Source: CAD feature listing. Evaluate the final solid. Frame: model axes, mm. Face numbers are marked on the shaded views. A direction names the side the tool comes from. Coordinates: 2 decimals unless noted, no trailing zeros. Write each loop counter-clockwise with the first axis right and the second up, starting at its lowest first coordinate (ties: lowest second). Pieces come first, ordered by that corner, then holes. Notation, with made-up numbers: M -28.75,81 L -21.75,81 A20 cw -21.75,89 Z; hole C 85,-35 d8. An arc over 180 degrees is marked long. One line per item, written item: value. Start each with the question number.
Item 1: Cut plane A-A, the plane z = 8. Output: boundary loops of the cut face in (x, y).
Item 2: Mould query, pull axis Z, two halves, no side actions, for the marked faces 3, 4 and 5. Classes: released by +Z, released by -Z, zero draft, split by the parting line, or undercut.
Item 3: Cut plane D-D, the plane z = 30. Output: boundary loops of the cut face in (x, y), then the cut area to 3 significant figures.
Item 4: Cut plane C-C, the plane y = 1.75. Output: boundary loops of the cut face in (x, z), then the cut area to 3 significant figures.
Item 5: Cut plane B-B, the plane x = 64. Output: boundary loops of the cut face in (y, z), then the cut area to 3 significant figures.
Item 6: Set-up query: the marked faces 1 and 2. Return all of +Z, -Z, +X, -X, +Y, -Y with unobstructed straight access to the full face (end or side cutting, diameter ignored); none if empty.
Item 7: Pin query (flat end, axial travel): P1, Ø6, axis at x = 19, z = 32, coming from the +Y side; P2, Ø8, axis at x = 6, z = 8, coming from the -Y side; P3, Ø1, axis at x = 26, y = 3.5, coming from the +Z side. Return the tip coordinate at first contact, or that it passes through.
Item 8: Ray query, L1, parallel to Z at x = 6, y = 4.5; L2, parallel to X at y = 0.5, z = 10; L3, parallel to Z at x = 8, y = 1. Return the intervals inside material, ascending. Write a range as from..to.
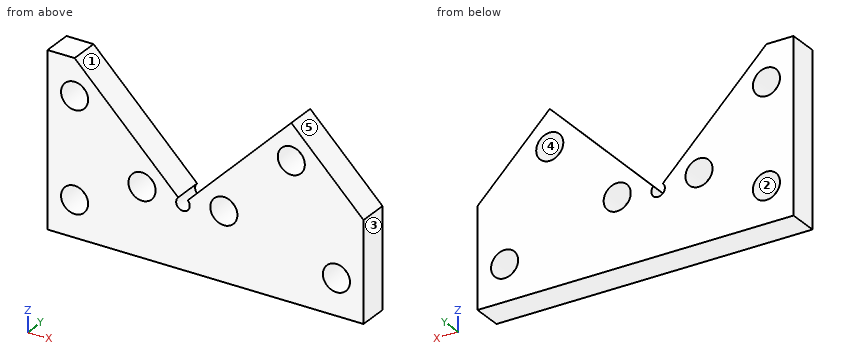
```python
from build123d import *

# Parameters (mm, degrees)
F0_R     = 3
F1_DEPTH = 6.6


with BuildPart() as f1:
    # F0 (on Front) → F1 (new body)
    with BuildSketch(Plane.XZ):
        with BuildLine():
            Line((0, 38), (0, 0))
            Line((0, 0), (70, 0))
            Line((70, 0), (70, 21.999999))
            Line((70, 21.999999), (54, 38))
            Line((54, 38), (31.060658, 15.06066))
            ThreePointArc((31.060658, 15.06066), (29.999998, 12.5), (28.939338, 15.06066))
            Line((28.939338, 15.06066), (6, 38))
            Line((6, 38), (0, 38))
        make_face()
        with Locations((6, 8)):
            Circle(F0_R, mode=Mode.SUBTRACT)
        with Locations((20.939338, 15.060661)):
            Circle(F0_R, mode=Mode.SUBTRACT)
        with Locations((64, 8)):
            Circle(F0_R, mode=Mode.SUBTRACT)
        with Locations((39.060658, 15.060661)):
            Circle(F0_R, mode=Mode.SUBTRACT)
        with Locations((6, 30)):
            Circle(F0_R, mode=Mode.SUBTRACT)
        with Locations((53.999996, 30)):
            Circle(F0_R, mode=Mode.SUBTRACT)
    extrude(amount=-F1_DEPTH)


solid = f1.part
```
From the geometry:
1. outline: M 0,0 L 3,0 L 3,6.6 L 0,6.6 Z; M 9,0 L 61,0 L 61,6.6 L 9,6.6 Z; M 67,0 L 70,0 L 70,6.6 L 67,6.6 Z
2. face 3: zero draft
2. face 4: undercut
2. face 5: released by +Z
3. outline: M 0,0 L 3,0 L 3,6.6 L 0,6.6 Z; M 9,0 L 14,0 L 14,6.6 L 9,6.6 Z; M 46,0 L 51,0 L 51,6.6 L 46,6.6 Z; M 57,0 L 62,0 L 62,6.6 L 57,6.6 Z
3. area: 119 mm²
4. outline: M 0,0 L 70,0 L 70,22 L 54,38 L 31.06,15.06 A1.5 cw long 28.94,15.06 L 6,38 L 0,38 Z; hole C 6,8 d6; hole C 6,30 d6; hole C 20.94,15.06 d6; hole C 39.06,15.06 d6; hole C 54,30 d6; hole C 64,8 d6
4. area: 1,780 mm²
5. outline: M 0,0 L 6.6,0 L 6.6,5 L 0,5 Z; M 0,11 L 6.6,11 L 6.6,28 L 0,28 Z
5. area: 145 mm²
6. face 1: +Z, +Y, -Y
6. face 2: +Y, -Y
7. P1: passes through
7. P2: stops at y = 0
7. P3: stops at z = 18.5
8. L1: z = 0..5, 11..27, 33..38
8. L2: x = 0..3.76, 8.24..61.76, 66.24..70
8. L3: z = 0..5.76, 10.24..27.76, 32.24..36
